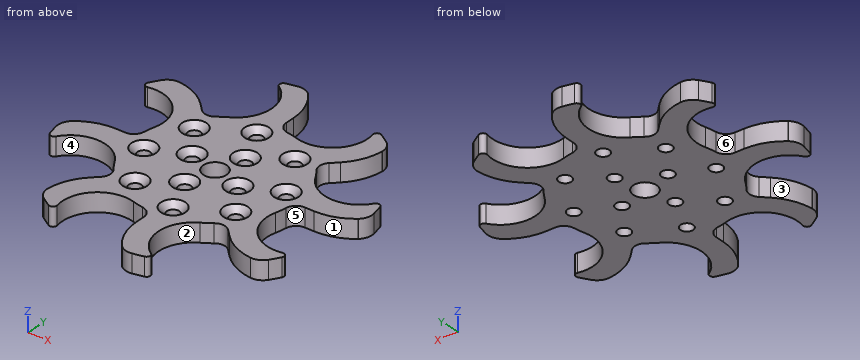
```python
from build123d import *

# Parameters (mm, degrees)
EXTRUDE_1_DEPTH           = 5
PATTERN_CIRCULAR_1_COUNT  = 8
FILLET_1_R                = 3
SKETCH_4_R                = 1.6
SKETCH_4_R_2              = 1.65
SKETCH_4_R_3              = 3.15
CUT_EXTRUDE_2_DEPTH       = 5
HOLE_WIZARD_1_D           = 3.4
HOLE_WIZARD_1_CSINK_D     = 6.6
HOLE_WIZARD_1_CSINK_ANGLE = 90


with BuildPart() as part:
    # 草图1 → 凸台-拉伸1 (new body)
    with BuildSketch(Plane.XY):
        with BuildLine():
            ThreePointArc((-10.356244554, 34.83376316), (-6.00280003, 26.616152007), (-10.75, 18.619546181))
            ThreePointArc((-10.75, 18.619546181), (5.56460947, -20.767405265), (0, 21.5))
            Line((0, 21.5), (0, 26.721510215))
            ThreePointArc((0, 26.721510215), (-0.876562566, 31.680090761), (-3.4, 36.037629801))
            ThreePointArc((-3.4, 36.037629801), (-3.429921119, 36.072346995), (-3.460629906, 36.106369449))
            ThreePointArc((-3.460629906, 36.106369449), (-5.148861305, 37.192002716), (-7.15188578, 37.320912767))
            ThreePointArc((-7.15188578, 37.320912767), (-8.622723673, 37.00876432), (-10.080061386, 36.638673044))
            ThreePointArc((-10.080061386, 36.638673044), (-10.803291061, 35.82575459), (-10.356244554, 34.83376316))
        make_face()
    extrude_1 = extrude(amount=EXTRUDE_1_DEPTH)

    # 阵列(圆周)1: 凸台-拉伸1 ×8 about axis
    pattern_circular_1_axis = Axis((0, 0, 0), (0, 0, 1))
    for i in range(1, PATTERN_CIRCULAR_1_COUNT):
        add(extrude_1.rotate(pattern_circular_1_axis, i * 360 / PATTERN_CIRCULAR_1_COUNT))

    # 圆角1
    fillet_1_edges = [part.edges().sort_by_distance(p)[0] for p in [
        (0, 21.5, 2.5),
        (-15.202795796, 15.202795796, 2.5),
        (-15.202795796, -15.202795796, 2.5),
        (15.202795796, -15.202795796, 2.5),
        (15.202795796, 15.202795796, 2.5),
        (21.5, 0, 2.5),
        (0, -21.5, 2.5),
        (-21.5, 0, 2.5),
    ]]
    fillet(fillet_1_edges, radius=FILLET_1_R)

    # 草图4 → 切除-拉伸2 (cut)
    with BuildSketch(Plane.XY.offset(5)):
        with Locations((-2.435529267, 17.329691203)):
            Circle(SKETCH_4_R)
        with Locations((10.531762905, 13.976121426)):
            Circle(SKETCH_4_R)
        with Locations((17.329691203, 2.435529267)):
            Circle(SKETCH_4_R)
        with Locations((13.976121426, -10.531762905)):
            Circle(SKETCH_4_R)
        with Locations((2.435529267, -17.329691203)):
            Circle(SKETCH_4_R)
        with Locations((-10.531762905, -13.976121426)):
            Circle(SKETCH_4_R)
        with Locations((-17.329691203, -2.435529267)):
            Circle(SKETCH_4_R)
        with Locations((-13.976121426, 10.531762905)):
            Circle(SKETCH_4_R)
        with Locations((2.015559033, 7.793588505)):
            Circle(SKETCH_4_R_2)
        with Locations((7.793588505, -2.015559033)):
            Circle(SKETCH_4_R_2)
        with Locations((-2.015559033, -7.793588505)):
            Circle(SKETCH_4_R_2)
        with Locations((-7.793588505, 2.015559033)):
            Circle(SKETCH_4_R_2)
        Circle(SKETCH_4_R_3)
    extrude(amount=-CUT_EXTRUDE_2_DEPTH, mode=Mode.SUBTRACT)

    # 打孔尺寸(%根据十字)槽半沉头木螺钉的类型1 (through all)
    with Locations(Plane(origin=(-13.976121426, 10.531762905, 5), x_dir=(1, 0, 0), z_dir=(0, 0, 1))):
        with Locations((0, 0), (11.540592159, 6.797928298), (24.507884331, 3.444358521), (31.305812629, -8.096233638), (27.952242852, -21.06352581), (16.411650693, -27.861454108), (3.444358521, -24.507884331), (-3.353569777, -12.967292172), (6.182532921, -8.516203872), (15.991680459, -2.7381744), (21.769709931, -12.547321938), (11.960562393, -18.32535141)):
            CounterSinkHole(HOLE_WIZARD_1_D / 2, HOLE_WIZARD_1_CSINK_D / 2, counter_sink_angle=HOLE_WIZARD_1_CSINK_ANGLE)


solid = part.part
```
Part model, mm, in its own coordinate system. Face numbers are marked on the shaded views. A direction names the side the tool comes from. Round coordinates to 2 decimals unless told otherwise and drop trailing zeros. Write each loop counter-clockwise with the first axis right and the second up, starting at its lowest first coordinate (ties: lowest second). Pieces come first, ordered by that corner, then holes. Notation, with made-up numbers: (-5, -20) -> (50, -20) arc R21 cw to (50, 3) -> close; hole circle Ø6 at (-20.5, -34.75). An arc over 180 degrees is marked (long way). Return JSON: item names as keys, results as strings. Group by question number.
Q1. Probe L1, parallel to X at y = -10, z = 2.35; L2, parallel to Y at x = 11, z = 3.2; L3, parallel to X at y = -13, z = 2.5. List the from-to ranges inside material, lowest first. Write a range as [from, to].
Q2. Saw through at A-A on y = 29. Write the cut outline in (x, z).
Q3. Mould opens along X. For the marked faces 1, 2 and 3 say: pulls with the +X half, pulls with the -X half, needs draft (parallel to the pull), parting line crosses it, or undercut.
Q4. Saw through at B-B on z = 1. State how many separate pieces and enclosed holes the cut face has, plus the area to 3 significant figures.
Q5. Pin check, flat tips, straight feed: pin 1 (5.5 mm diameter, centred on x = -13.98, y = 10.53, fed in from -Z); pin 2 (4 mm diameter, centred on x = -2.02, y = -7.79, fed in from +Z); pin 3 (2.5 mm diameter, centred on x = -25.5, z = 3, fed in from +Y); pin 4 (1.2 mm diameter, centred on x = 25.5, z = 2, fed in from -Y). Stop position of each tip, or through.
Q6. Which spindle directions (+Z, -Z, +X, -X, +Y, -Y) get a long thin tool onto all of the face, cutting with end or side? Do the marked faces 4, 5 and 6. Say none if no direction does.
Answer:
{
 "1": {"L1": "[-36.66, -34.59], [-19.1, 12.36], [15.59, 20.65]", "L2": "[-18.47, 12.34], [15.61, 20.92]", "L3": "[-17.12, -11.92], [-9.14, 21.85]"},
 "2": {"outline": "(-6.25, 0) -> (-0.18, 0) -> (-0.18, 5) -> (-6.25, 5) -> close; (17.48, 0) -> (22.99, 0) -> (22.99, 5) -> (17.48, 5) -> close"},
 "3": {"face 1": "pulls with the +X half", "face 2": "undercut", "face 3": "pulls with the -X half"},
 "4": {"separate pieces": "1", "enclosed holes": "13", "area": "2,190 mm2"},
 "5": {"pin 1": "z = 0", "pin 2": "z = 3.71", "pin 3": "y = 22.94", "pin 4": "y = -22.81"},
 "6": {"face 4": "+Z, -Z", "face 5": "+Z, -Z, +X", "face 6": "+Z, -Z, -X"}
}
